Model file for the job. Use its own axes, mm. A direction names the side the tool comes from. Round coordinates to 2 decimals unless told otherwise and drop trailing zeros. Order: outer loops, then holes, each group sorted by start corner. A loop starts at its lowest first (then second) coordinate and runs counter-clockwise, first axis right, second up. Notation, with made-up numbers: (-5.75, 58.5) - (4.25, 58.5) arc R5 ccw to (4.25, 67.5) - close; hole circle Ø6 at (-25, -32.75). An arc over 180 degrees is marked (long way). Put each result on its own line as item: value. Start each with the question number.
Item 1: Which spindle directions (+Z, -Z, +X, -X, +Y, -Y) get a long thin tool onto all of the face, cutting with end or side? Do faces 1 (the face through (-1000, 40, 507)), 2 (the face through (-25.4, 93, 507)), 3 (the face through (-987, 80.4, 507)). Say none if no direction does.
Item 2: Probe probe 1 along Z at (x, y) = (-638, 49.5); probe 2 along X at (y, z) = (35.5, 877.5); probe 3 along Y at (x, z) = (-194.5, 717). List the from-to ranges inside material, lowest first.
Item 3: Saw through at B-B on x = -156. List the corners of the cut face in (y, z).
Item 4: Mould opens along Z. For faces 4 (the face through (-974.6, 38, 493)), 5 (the face through (-493, 53, -25.4)), 6 (the face through (-507, 53, 1025.4)), 7 (the face through (-16, 105.4, 502)) say: pulls with the +Z half, pulls with the -Z half, needs draft (parallel to the pull), parting line crosses it, or undercut.
Item 5: Saw through at A-A on z = 709. List the corners of the cut face in (x, y), plus the area to 3 significant figures.
Item 6: Pin check, flat tip, straight feed: pin 1 Ø5 at (x, z) = (-300.5, 200) entering from +Y. Stop position of the tip, or through.
Autodesk Inventor part; units mm, degrees
ref_plane "Work Plane1" through (-1000, 65.4, 1000) normal (0, 1, 0) x (1, 0, 0)
ref_plane "Work Plane2" through (-1000, 0, 500) normal (0, 0, 1) x (1, 0, 0)
ref_plane "Work Plane3" through (0, 0, 1025.4) normal (1, 0, 0) x (0, 0, -1)
sketch "Sketch1" plane through (0, 0, 0) normal (0, 1, 0) x (-1, 0, 0)
  line L0 (0, 0) -> (1000, 0)
  line L1 (1000, 0) -> (1000, 1000)
  line L2 (1000, 1000) -> (0, 1000)
  line L3 (0, 1000) -> (0, 0)
  dimension "d0" = 1000
  dimension "d1" = 1000
extrude "Extrusion1" add sketch "Sketch1" along normal blind 25.4
sketch "Sketch2" plane through (0, 0, 0) normal (1, 0, 0) x (0, 1, 0)
  line L0 (25.4, 1000) -> (25.4, 0)
  line L1 (25.4, 0) -> (105.4, 0)
  line L2 (105.4, 0) -> (105.4, 1000)
  line L3 (105.4, 1000) -> (25.4, 1000)
  line L4 (25.4, 1000) -> (25.4, 0)
  point P0 (0, 0)
  dimension "d4" = 80
  dimension "d5" = 1000
extrude "Extrusion2" add sketch "Sketch2" against normal blind 25.4
sketch "Sketch3" plane through (-1000, 0, 0) normal (-1, 0, 0) x (0, 0, 1)
  line L0 (1000, 0) -> (1000, 25.4)
  line L1 (1000, 105.4) -> (0, 105.4)
  line L2 (1000, 25.4) -> (0, 25.4)
  line L3 (0, 25.4) -> (0, 105.4)
  line L4 (0, 105.4) -> (1000, 105.4)
  line L5 (1000, 105.4) -> (1000, 25.4)
  point P0 (0, 0)
  dimension "d8" = 1000
  dimension "d9" = 80
extrude "Extrusion3" add sketch "Sketch3" against normal blind 25.4
sketch "Sketch4" plane through (-25.4, 0, 0) normal (-1, 0, 0) x (0, 0, 1)
  line L0 (0, 50.4) -> (1000, 50.4)
  line L1 (1000, 50.4) -> (1000, 80.4)
  line L2 (1000, 80.4) -> (0, 80.4)
  line L3 (0, 80.4) -> (0, 50.4)
  point P0 (0, 0)
  dimension "d12" = 1000
  dimension "d13" = 30
extrude "Extrusion4" cut sketch "Sketch4" against normal blind 25.4
sketch "Sketch5" plane through (-974.6, 0, 0) normal (1, 0, 0) x (0, 0, -1)
  line L0 (0, 25.4) -> (0, 105.4)
  line L1 (0, 50.4) -> (-1000, 50.4)
  line L2 (-1000, 50.4) -> (-1000, 80.4)
  line L3 (-1000, 80.4) -> (0, 80.4)
  line L4 (0, 80.4) -> (0, 50.4)
  line L5 (0, 25.4) -> (-1000, 25.4)
  point P0 (0, 0)
  point P1 (0, 80.4)
  dimension "d16" = 1000
  dimension "d17" = 30
  dimension "d18" = 25
extrude "Extrusion5" cut sketch "Sketch5" against normal blind 25.4
ref_plane "Work Plane1" through (-1000, 65.4, 1000) normal (0, 1, 0) x (1, 0, 0)
sketch "Sketch6" plane through (-1000, 0, 1000) normal (0, 0, 1) x (1, 0, 0)
  line L0 (0, 80.4) -> (0, 105.4)
  line L1 (1000, 0) -> (0, 0)
  line L2 (0, 0) -> (0, 105.4)
  line L3 (0, 105.4) -> (1000, 105.4)
  line L4 (1000, 105.4) -> (1000, 0)
extrude "Extrusion6" add sketch "Sketch6" along normal blind 25.4
sketch "Sketch7" plane through (0, 0, 0) normal (0, 0, -1) x (-1, 0, 0)
  line L0 (0, 105.4) -> (1000, 105.4)
  line L1 (0, 0) -> (1000, 0)
  line L2 (1000, 0) -> (1000, 105.4)
  line L3 (1000, 105.4) -> (0, 105.4)
  line L4 (0, 105.4) -> (0, 0)
extrude "Extrusion7" add sketch "Sketch7" along normal blind 25.4
ref_plane "Work Plane2" through (-1000, 0, 500) normal (0, 0, 1) x (1, 0, 0)
ref_plane "Work Plane3" through (0, 0, 1025.4) normal (1, 0, 0) x (0, 0, -1)
properties material "Iron, Cast"
Results found:
1. face 1: +Z, -Z, -X, +Y, -Y
1. face 2: +Y
1. face 3: +X, -X
2. probe 1: z = -25.4 to 0, 1000 to 1025.4
2. probe 2: x = -1000 to -974.6, -25.4 to 0
2. probe 3: y = 0 to 25.4
3. outline: (0, -25.4) - (105.4, -25.4) - (105.4, 0) - (25.4, 0) - (25.4, 1000) - (105.4, 1000) - (105.4, 1025.4) - (0, 1025.4) - close
4. face 4: undercut
4. face 5: pulls with the -Z half
4. face 6: pulls with the +Z half
4. face 7: needs draft
5. outline: (-1000, 0) - (0, 0) - (0, 50.4) - (-25.4, 50.4) - (-25.4, 25.4) - (-974.6, 25.4) - (-974.6, 50.4) - (-1000, 50.4) - close; (-1000, 80.4) - (-974.6, 80.4) - (-974.6, 105.4) - (-1000, 105.4) - close; (-25.4, 80.4) - (0, 80.4) - (0, 105.4) - (-25.4, 105.4) - close
5. area: 27,900 mm²
6. pin 1: stops at y = 25.4
